Verification items for the finished model (mm, model axes). A direction names the side the tool comes from. Round coordinates to 2 decimals unless told otherwise and drop trailing zeros. Write each loop counter-clockwise with the first axis right and the second up, starting at its lowest first coordinate (ties: lowest second). Pieces come first, ordered by that corner, then holes. Notation, with made-up numbers: M 79.5,66 L 119.5,66 A33 cw 119.5,103 Z; hole C 20.5,7.25 d9. An arc over 180 degrees is marked long. One line per item, written item: value. Start each with the question number.
from build123d import *

# Parameters (mm, degrees)
STOCK_COMPARTMENT_START            = 0.33
STOCK_COMPARTMENT_BOTTOM_1_DEPTH   = 2
STOCK_COMPARTMENT_START_2          = -2.3
STOCK_COMPARTMENT_BOTTOM_1_2_DEPTH = 2.63
BOSS_EXTRUDE1_START                = -2
BOSS_EXTRUDE1_DEPTH                = 2


# Read off the part's stored shape, not the designer's step: Stock-Compartment Bottom-1
with BuildPart() as part:
    # Stock-Compartment Bottom-1 outline → Stock-Compartment Bottom-1 (new body)
    with BuildSketch(Plane(origin=(0, 0, 0), x_dir=(1, 0, 0), z_dir=(0, 1, 0)).offset(STOCK_COMPARTMENT_START)):
        with BuildLine():
            Line((24.5, -5.716120649), (24.5, 8.453194282))
            Line((24.5, 8.453194282), (-24.5, 8.453194282))
            Line((-24.5, 8.453194282), (-24.5, -5.716120649))
            ThreePointArc((-24.5, -5.716120649), (-20.163977484, -11.042600894), (-14.696938457, -15.2))
            Line((-14.696938457, -15.2), (14.696938457, -15.2))
            ThreePointArc((14.696938457, -15.2), (20.163977484, -11.042600894), (24.5, -5.716120649))
        make_face()
    extrude(amount=STOCK_COMPARTMENT_BOTTOM_1_DEPTH)

    # Stock-Compartment Bottom-1 2 outline → Stock-Compartment Bottom-1 2 (add)
    with BuildSketch(Plane(origin=(0, 0, 0), x_dir=(1, 0, 0), z_dir=(0, 1, 0)).offset(STOCK_COMPARTMENT_START_2)):
        with BuildLine():
            Line((24.5, -5.716120649), (24.5, -1.546805718))
            ThreePointArc((24.5, -1.546805718), (20.180507814, -8.137310399), (14.142135624, -13.2))
            Line((14.142135624, -13.2), (-14.142135624, -13.2))
            ThreePointArc((-14.142135624, -13.2), (-20.180507814, -8.137310399), (-24.5, -1.546805718))
            Line((-24.5, -1.546805718), (-24.5, -5.716120649))
            ThreePointArc((-24.5, -5.716120649), (-20.163977484, -11.042600894), (-14.696938457, -15.2))
            Line((-14.696938457, -15.2), (14.696938457, -15.2))
            ThreePointArc((14.696938457, -15.2), (20.163977484, -11.042600894), (24.5, -5.716120649))
        make_face()
    extrude(amount=STOCK_COMPARTMENT_BOTTOM_1_2_DEPTH)

    # Sketch1 → Boss-Extrude1 (add)
    with BuildSketch(Plane(origin=(0, 2.33, 0), x_dir=(1, 0, 0), z_dir=(0, 1, 0)).offset(BOSS_EXTRUDE1_START)):
        with BuildLine():
            Line((-25.7, 33.453194282), (-25.7, 8.453194282))
            Line((-25.7, 8.453194282), (-25.7, -3.635400999))
            ThreePointArc((-25.7, -3.635400999), (-25.121551476, -4.688190068), (-24.5, -5.716120649))
            Line((-24.5, -5.716120649), (-24.5, 8.453194282))
            Line((-24.5, 8.453194282), (24.5, 8.453194282))
            Line((24.5, 8.453194282), (24.5, -5.716120649))
            ThreePointArc((24.5, -5.716120649), (25.121551476, -4.688190068), (25.7, -3.635400999))
            Line((25.7, -3.635400999), (25.7, 8.453194282))
            Line((25.7, 8.453194282), (25.7, 33.453194282))
            Line((25.7, 33.453194282), (-25.7, 33.453194282))
        make_face()
    extrude(amount=BOSS_EXTRUDE1_DEPTH)


solid = part.part
1) Thickness scan on line 1 (Z direction, x = -4, y = 0.05); line 2 (Y direction, x = 23, z = -29.5); line 3 (X direction, y = -1.5, z = 4). Record the ranges inside material, lowest first.
2) Cross-section at C-C (x = 2). Record the boundary of the cut face in (y, z).
3) Cross-section at D-D (x = 18). Record the boundary of the cut face in (y, z).
4) Access from +Z, -Z, +X, -X, +Y, -Y to the whole of each face (thin tool, end or side, straight path). Record for faces 5 (the flat face through (-24.5, -1, 4)), 6 (the cylindrical face through (-20.107, -1.003, 8.22)), 7 (the flat face through (24.5, -1, 4)).
5) Cross-section at B-B (z = -23). Record the boundary of the cut face in (x, y), then the cut area to 3 significant figures.
6) Mould release check, pull along X, two halves, no side actions. Record for faces 1 (the flat face through (-0.1, -2.3, 13.4)), 2 (the flat face through (-25.7, 1, -15)), 3 (the cylindrical face through (20.254, -1.003, 8.054)), 4 (the flat face through (0, -1, 13.2)): pulls with the +X half, pulls with the -X half, needs draft (parallel to the pull), parting line crosses it, or undercut.
7) Gauge pin test, flat ends, axial feed: pin 1 Ø2 at (y, z) = (1, 7) entering from +X; pin 2 Ø1 at (x, y) = (18, -1) entering from +Z; pin 3 Ø2 at (x, y) = (-5, -1) entering from -Z. Record the tip position at first contact, or that the pin passes through.
8) Cross-section at A-A (y = 1.1). Record the boundary of the cut face in (x, z).
Results below:
1. line 1: z = 13.2 to 15.2
1. line 2: y = 0.33 to 2.33
1. line 3: x = -24.5 to -23.21, 23.21 to 24.5
2. outline: M -2.3,13.2 L 0.33,13.2 L 0.33,-33.45 L 2.33,-33.45 L 2.33,15.2 L -2.3,15.2 Z
3. outline: M -2.3,10.32 L 0.33,10.32 L 0.33,-33.45 L 2.33,-33.45 L 2.33,12.94 L -2.3,12.94 Z
4. face 5: +Z, -Z, -X, -Y
4. face 6: -Z, -Y
4. face 7: +Z, -Z, +X, -Y
5. outline: M -25.7,0.33 L 25.7,0.33 L 25.7,2.33 L -25.7,2.33 Z
5. area: 103 mm²
6. face 1: needs draft
6. face 2: pulls with the -X half
6. face 3: undercut
6. face 4: undercut
7. pin 1: stops at x = 24.32
7. pin 2: stops at z = 13.32
7. pin 3: stops at z = 13.2
8. outline: M -25.7,-33.45 L 25.7,-33.45 L 25.7,3.64 A29 ccw 14.7,15.2 L -14.7,15.2 A29 ccw -25.7,3.64 Z
